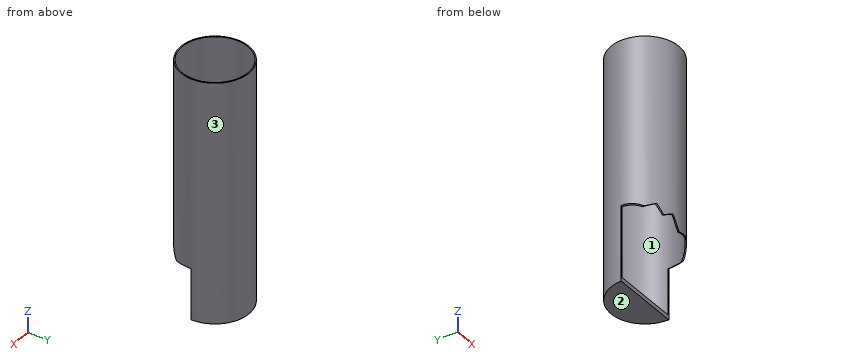
```python
from build123d import *

# Parameters (mm, degrees)
F0_R     = 203.2
F0_R_2   = 196.85
F1_DEPTH = 1438.656
F2_R     = 196.85
F3_DEPTH = 25.4
F5_DEPTH = 508


with BuildPart() as f1:
    # F0 (on Top) → F1 (new body)
    with BuildSketch(Plane.XY):
        Circle(F0_R)
        Circle(F0_R_2, mode=Mode.SUBTRACT)
    extrude(amount=F1_DEPTH)

    # F2 (on face) → F3 (join)
    with BuildSketch(Plane(origin=(0, 0, 0), x_dir=(1, 0, 0), z_dir=(0, 0, -1))):
        Circle(F2_R)
    extrude(amount=-F3_DEPTH)

    # F4 (on Front) → F5 (cut)
    with BuildSketch(Plane.XZ):
        Polygon((-233.4638088942, 475.3084182739), (-262.1978223324, -27.536733076), (319.6658492088, -27.536733076), (319.6658492088, 288.5373830795), (228.6748290062, 317.2713816166), (171.2068021297, 288.5373830795), (94.5827811956, 355.5833995342), (0, 329.2438983917), (-44.2982390523, 413.0514264107), (-95.6870245125, 385.8887984614), (-126.9621838043, 445.0580531478), (-167.1748505567, 423.8027987949), align=None)
    extrude(amount=F5_DEPTH, mode=Mode.SUBTRACT)


solid = f1.part
```
For this review, take the finished solid that the model builds, in its own axes (mm). Face numbers are marked on the shaded views. Give positions to 0.01 mm unless a question says otherwise; leave off trailing zeros. Write each loop counter-clockwise with the first axis right and the second up, starting at its lowest first coordinate (ties: lowest second). Pieces come first, ordered by that corner, then holes.
Item 1: Take a section at B-B (y = 166.5). Give the boundary of the cut face in (x, z), and give its area (3 significant figures).
Item 2: Wall thickness on probe 1 along Y at (x, z) = (0, 420); probe 2 along Y at (x, z) = (-9, 1295.5): over which ranges is each line inside the solid? List them lowest first.
Item 3: Take a section at A-A (z = 1061.5). Give the boundary of the cut face in (x, y), and give its area (3 significant figures).
Item 4: Take a section at D-D (y = 64). Give the boundary of the cut face in (x, z), and give its area (3 significant figures).
Item 5: The part is to be moulded in two halves that separate along Y. For the marked faces 1, 2 and 3, say which applies: +Y half, -Y half, draft (parallel to the pull), parting line (faces both ways), or undercut.
Item 6: Insertion check: P1, Ø4, axis at y = 37, z = 459, coming from the +X side; P2, Ø5, axis at x = 125, z = 1027.5, coming from the +Y side; P3, Ø8, axis at x = -23, z = 290, coming from the +Y side. Each pin has a flat end and moves straight along its axis. Give the tip position at first contact, or say it passes through.
Item 7: Take a section at C-C (z = 136). Give the boundary of the cut face in (x, y), and give its area (3 significant figures).
Established:
1. outline: (-116.48, 0) - (116.48, 0) - (116.48, 1438.66) - (105.01, 1438.66) - (105.01, 25.4) - (-105.01, 25.4) - (-105.01, 1438.66) - (-116.48, 1438.66) - close
1. area: 38,300 mm2
2. probe 1: y = -203.2 to -196.85, 196.85 to 203.2
2. probe 2: y = -203 to -196.64, 196.64 to 203
3. outline: circle Ø406.4 at (0, 0); hole circle Ø393.7 at (0, 0)
3. area: 7,980 mm2
4. outline: (-192.86, 0) - (192.86, 0) - (192.86, 1438.66) - (186.16, 1438.66) - (186.16, 25.4) - (-186.16, 25.4) - (-186.16, 1438.66) - (-192.86, 1438.66) - close
4. area: 28,700 mm2
5. face 1: undercut
5. face 2: draft
5. face 3: parting line
6. P1: stops at x = 200.16
6. P2: stops at y = 162.12
6. P3: stops at y = 202.31
7. outline: (-203.2, 0) - (-196.85, 0) arc R196.85 cw to (196.85, 0) - (203.2, 0) arc R203.2 ccw to start
7. area: 3,990 mm2
